Design review of the part built by this model. Coordinates are the model's own, in mm. Face numbers are marked on the shaded views. A direction names the side the tool comes from. Coordinates: 2 decimals unless noted, no trailing zeros. Write each loop counter-clockwise with the first axis right and the second up, starting at its lowest first coordinate (ties: lowest second). Pieces come first, ordered by that corner, then holes. Notation, with made-up numbers: (-35.5, 82) -> (-3.5, 82) arc R27 ccw to (-3.5, 118) -> close; hole circle Ø2 at (62, -39.5). An arc over 180 degrees is marked (long way). One line per question, with ' | ' between items. Start each with the question number.
Q1. For P1, Ø1.4, axis at x = 13, y = 2, coming from the +Z side; P2, Ø3.5, axis at x = 13, y = 5, coming from the -Z side, all flat-tipped, find the tip position at first contact; note any pin that passes through.
Q2. Wall thickness on probe 1 along Y at (x, z) = (13, -2.05); probe 2 along Y at (x, z) = (13.25, -0.3); probe 3 along X at (y, z) = (4.75, -2): over which ranges is each line inside the solid? List them lowest first.
Q3. Add section A-A on y = 2. State the section outline as (x, z) points.
Q4. Add section D-D on z = -2.45. State the section outline as (x, y) points, and give its area (3 significant figures).
Q5. Add section C-C on y = 7. State the section outline as (x, z) points, and give its area (3 significant figures).
Q6. Add section B-B on x = 13. State the section outline as (y, z) points, and give its area (3 significant figures).
Q7. Draft analysis for pull direction Y (two halves, no side actions). For the marked faces 3, 4 and 5, state which applies: pulls with the +Y half, pulls with the -Y half, needs draft (parallel to the pull), parting line crosses it, or undercut.
Q8. For the marked faces 1 and 2, list the 3-axis set-ups (+Z, -Z, +X, -X, +Y, -Y) from which the entire face can be reached by the end or side of a thin tool; tool diameter is ignored.
from build123d import *

# Parameters (mm, degrees)
SKETCH1_R           = 1
BOSS_EXTRUDE1_DEPTH = 10
SKETCH5_R           = 0.7
SKETCH5_R_2         = 0.8
SKETCH5_R_3         = 2
CUT_EXTRUDE3_DEPTH  = 23.681269806
SKETCH7_W           = 11
SKETCH7_H           = 15.934078747
CUT_EXTRUDE4_DEPTH  = 23.681269806


with BuildPart() as part:
    # Sketch1 → Boss-Extrude1 (new body)
    with BuildSketch(Plane(origin=(0, 0, 0), x_dir=(1, 0, 0), z_dir=(0, 1, 0))):
        Polygon((0, 0), (20, 0), (20, 5), (15.5, 5), (15.5, 3.8), (0, 3.8), align=None)
        with Locations(Location((2.5, 2, 0), (0, 0, 270))):
            Circle(SKETCH1_R, mode=Mode.SUBTRACT)
        with Locations(Location((17.5, 2, 0), (0, 0, 270))):
            Circle(SKETCH1_R, mode=Mode.SUBTRACT)
    extrude(amount=BOSS_EXTRUDE1_DEPTH)

    # Sketch5 → Cut-Extrude3 (cut, through all)
    with BuildSketch(Plane(origin=(0, 0, -3.8), x_dir=(-1, 0, 0), z_dir=(0, 0, -1))):
        with Locations((-13, 4.971794193)):
            Circle(SKETCH5_R)
        with Locations((-13, 8)):
            Circle(SKETCH5_R_2)
        with Locations((-6.5, 4)):
            Circle(SKETCH5_R_3)
        with Locations((-13, 2)):
            Circle(SKETCH5_R_2)
    extrude(amount=-CUT_EXTRUDE3_DEPTH, mode=Mode.SUBTRACT)

    # Sketch7 → Cut-Extrude4 (cut, through all)
    with BuildSketch(Plane(origin=(0, 0, -3.8), x_dir=(-1, 0, 0), z_dir=(0, 0, -1))):
        with Locations((-5.5, 5.758979145)):
            Rectangle(SKETCH7_W, SKETCH7_H)
    extrude(amount=-CUT_EXTRUDE4_DEPTH, mode=Mode.SUBTRACT)


solid = part.part
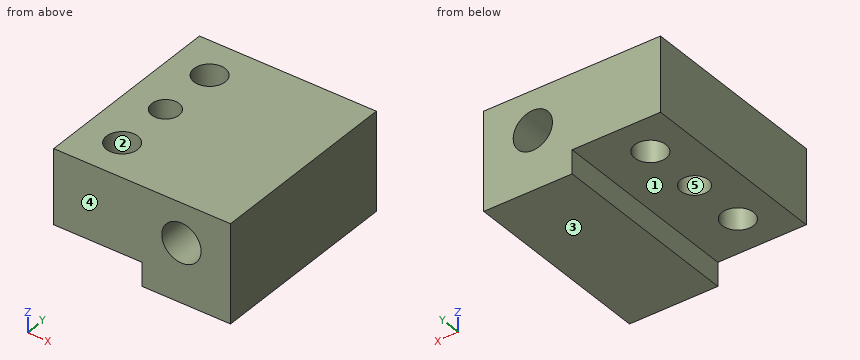
Output values:
1) P1: passes through | P2: stops at z = -3.8
2) probe 1: y = 0 to 1.2, 2.8 to 4.27, 5.67 to 7.2, 8.8 to 10 | probe 2: y = 0 to 1.24, 2.76 to 4.32, 5.63 to 7.24, 8.76 to 10 | probe 3: x = 11 to 12.34, 13.66 to 16.5, 18.5 to 20
3) outline: (11, -3.8) -> (12.2, -3.8) -> (12.2, 0) -> (11, 0) -> close; (13.8, -3.8) -> (15.5, -3.8) -> (15.5, -5) -> (20, -5) -> (20, 0) -> (13.8, 0) -> close; hole circle Ø2 at (17.5, -2)
4) outline: (11, 0) -> (16.61, 0) -> (16.61, 10) -> (11, 10) -> close; (18.39, 0) -> (20, 0) -> (20, 10) -> (18.39, 10) -> close; hole circle Ø1.6 at (13, 2); hole circle Ø1.6 at (13, 8); hole circle Ø1.4 at (13, 4.97) | area: 66.6 mm2
5) outline: (11, -3.8) -> (15.5, -3.8) -> (15.5, -5) -> (20, -5) -> (20, 0) -> (11, 0) -> close; hole circle Ø2 at (17.5, -2) | area: 36.5 mm2
6) outline: (0, -3.8) -> (1.2, -3.8) -> (1.2, 0) -> (0, 0) -> close; (2.8, -3.8) -> (4.27, -3.8) -> (4.27, 0) -> (2.8, 0) -> close; (5.67, -3.8) -> (7.2, -3.8) -> (7.2, 0) -> (5.67, 0) -> close; (8.8, -3.8) -> (10, -3.8) -> (10, 0) -> (8.8, 0) -> close | area: 20.5 mm2
7) face 3: needs draft | face 4: pulls with the -Y half | face 5: undercut
8) face 1: -Z, -X, +Y, -Y | face 2: +Z, -Z
